```python
from build123d import *

# Parameters (mm, degrees)
SFAZOWANIE2_SIZE = 3


with BuildPart() as part:
    # Szkic1 → Obrót1 (revolve)
    with BuildSketch(Plane.XY, mode=Mode.PRIVATE) as obr_t1_sk:
        Polygon((-122, 69.81557254), (-122, -10.18442746), (-50.745506493, -10.18442746), (-49, 89.81557254), (-85, 89.81557254), (-85, 84.81557254), (-107, 84.81557254), (-107, 69.81557254), align=None)
    revolve(obr_t1_sk.sketch.rotate(Axis((0, 0, 0), (0, 1, 0)), 270), axis=Axis((0, 0, 0), (0, 1, 0)))

    # Sfazowanie2
    sfazowanie2_edges = [part.edges().sort_by_distance(p)[0] for p in [
        (0, -10.18442746, 122),
        (0, 69.81557254, 122),
    ]]
    chamfer(sfazowanie2_edges, length=SFAZOWANIE2_SIZE)


solid = part.part
```
Input: part model. Units: mm. Frame: model coordinates. A direction names the side the tool comes from. Give positions to 0.01 mm unless a question says otherwise; leave off trailing zeros. Write each loop counter-clockwise with the first axis right and the second up, starting at its lowest first coordinate (ties: lowest second). Pieces come first, ordered by that corner, then holes. Notation, with made-up numbers: (38, 48.25) - (60, 48.25) arc R26 cw to (60, 77.25) - close; hole circle Ø7 at (-35, 52). An arc over 180 degrees is marked (long way). Write item = value, one per line. Start each with the question number.
1) Reachability of faces 4 (the face through (-80, 84.816, 31)), 5 (the face through (37, 89.816, 37)) from +Z, -Z, +X, -X, +Y, -Y: full face, straight path, thin tool, end or side. Return the list, or none.
2) Cut plane B-B (y = 49). Return loops of the section in (x, z), and give its area (3 significant figures).
3) Pin query (flat end, axial travel): pin 1 (2 mm diameter, centred on y = 69.5, z = -62, fed in from -X); pin 2 (1 mm diameter, centred on x = 55, z = 88, fed in from +Y); pin 3 (1.5 mm diameter, centred on y = 75.5, z = -3.5, fed in from +X). Return the tip coordinate at first contact, or that it passes through.
4) Cut plane A-A (y = 18). Return loops of the section in (x, z), and give its area (3 significant figures).
5) Material intervals for L1, parallel to X at y = 4, z = 0.5; L2, parallel to X at y = 68.5, z = 32.5; L3, parallel to Z at x = -17.5, y = 2.5, sorted ascending. Write a range as [from, to].
6) Draft query along Z for faces 1 (the face through (51.721, 87.281, 67.453)), 2 (the face through (-2, -10.184, -51)), 3 (the face through (-14.977, 40.516, -47.558)). Return one class per face: pulls with the +Z half, pulls with the -Z half, needs draft (parallel to the pull), parting line crosses it, or undercut.
Answers follow:
q1.face_4 = +Y
q1.face_5 = +Z, -Z, +X, -X, +Y
q2.outline = circle Ø244 at (0, 0); hole circle Ø99.42 at (0, 0)
q2.area = 39,000 mm^2
q3.pin_1 = -103.26
q3.pin_2 = 84.82
q3.pin_3 = 106.96
q4.outline = circle Ø244 at (0, 0); hole circle Ø100.51 at (0, 0)
q4.area = 38,800 mm^2
q5.L1 = [-122, -50.5], [50.5, 122]
q5.L2 = [-115.84, -37.17], [37.17, 115.84]
q5.L3 = [-120.74, -47.4], [47.4, 120.74]
q6.face_1 = parting line crosses it
q6.face_2 = needs draft
q6.face_3 = undercut
